Drawing for the job (mm, zero at the part's lowest x, y, z). A direction names the side the tool comes from. Coordinates: 2 decimals unless noted, no trailing zeros. Order: outer loops, then holes, each group sorted by start corner. A loop starts at its lowest first (then second) coordinate and runs counter-clockwise, first axis right, second up. Notation, with made-up numbers: M 86.25,51 L 113.25,51 A16 cw 113.25,58 Z; hole C 50,-28.75 d10. An arc over 180 degrees is marked long. Write item = value, one per line. Start each with the question number.
Q1. Band-saw the part on B-B on z = 9.5. Write the cut outline in (x, y), plus the area to 4 significant figures.
Q2. Band-saw the part on D-D on y = 39. Write the cut outline in (x, z).
Q3. 3-axis set-ups, long thin cutter, end or side, ignore diameter. For the marked faces 1 and 2: which of +Z, -Z, +X, -X, +Y, -Y reach the whole face in a straight line?
Q4. Drill centre lines: probe 1 along X at (y, z) = (3.9, 35); probe 2 along X at (y, z) = (2, 15); probe 3 along X at (y, z) = (41, 39.5). Where is each one in solid material? Low to high.
Q5. Band-saw the part on C-C on y = 53. Write the cut outline in (x, z).
Q6. Band-saw the part on A-A on x = 21. Write the cut outline in (y, z).
Q7. Pin check, flat tips, straight feed: P1, Ø2.5, axis at x = 37, z = 35, coming from the -Y side; P2, Ø8, axis at y = 37.5, z = 25, coming from the +X side; P3, Ø2, axis at y = 35, z = 6.5, coming from the +X side; P4, Ø4.5, axis at x = 37, z = 15, coming from the +Y side. Stop position of each tip, or through.
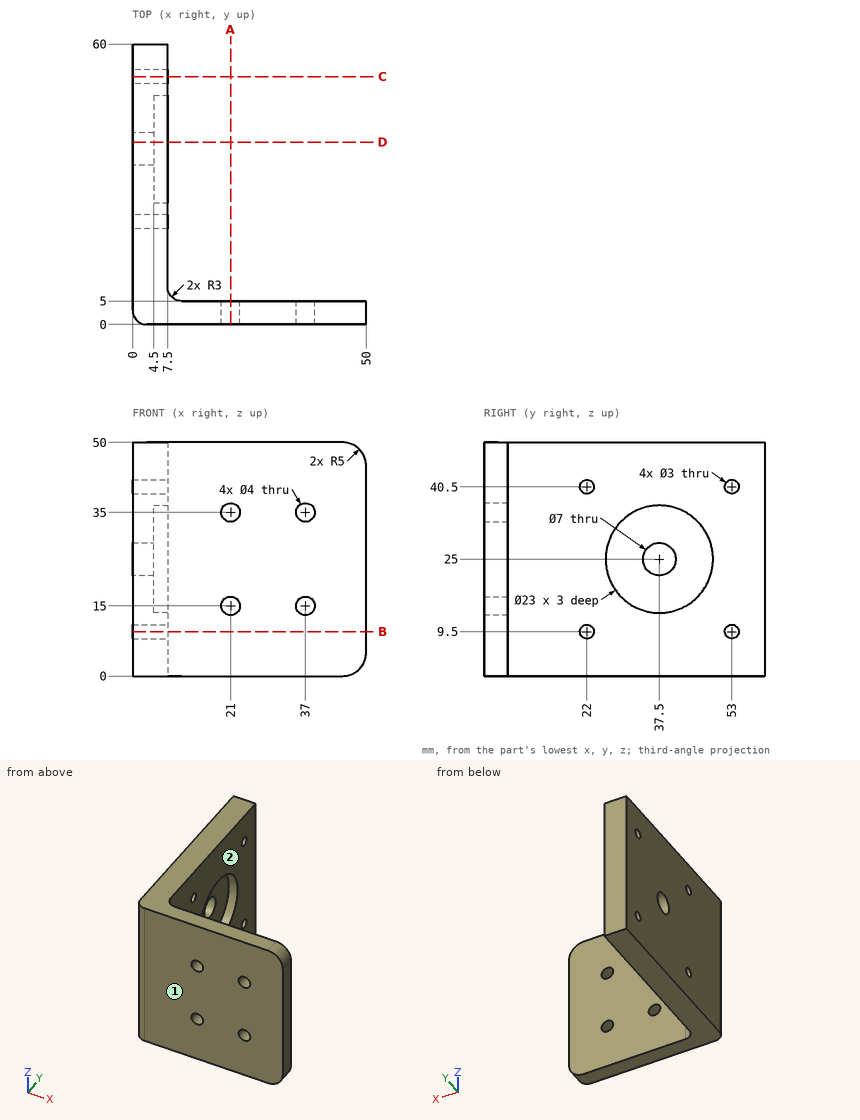
Recorded:
q1.outline = M 0,3 A3 ccw 3,0 L 50,0 L 50,5 L 10.5,5 A3 cw 7.5,8 L 7.5,20.5 L 0,20.5 Z; M 0,23.5 L 7.5,23.5 L 7.5,51.5 L 0,51.5 Z; M 0,54.5 L 7.5,54.5 L 7.5,60 L 0,60 Z
q1.area = 617.5 mm2
q2.outline = M 0,0 L 7.5,0 L 7.5,13.6 L 4.5,13.6 L 4.5,21.84 L 0,21.84 Z; M 0,28.16 L 4.5,28.16 L 4.5,36.4 L 7.5,36.4 L 7.5,50 L 0,50 Z
q3.face_1 = +Z, -Z, +X, -X, -Y
q3.face_2 = +Z, -Z, +X, +Y
q4.probe_1 = 0 to 19, 23 to 35, 39 to 50
q4.probe_2 = 0.17 to 19, 23 to 35, 39 to 50
q4.probe_3 = 0 to 7.5
q5.outline = M 0,0 L 7.5,0 L 7.5,8 L 0,8 Z; M 0,11 L 7.5,11 L 7.5,39 L 0,39 Z; M 0,42 L 7.5,42 L 7.5,50 L 0,50 Z
q6.outline = M 0,0 L 5,0 L 5,13 L 0,13 Z; M 0,17 L 5,17 L 5,33 L 0,33 Z; M 0,37 L 5,37 L 5,50 L 0,50 Z
q7.P1 = through
q7.P2 = 4.5
q7.P3 = 7.5
q7.P4 = 5
